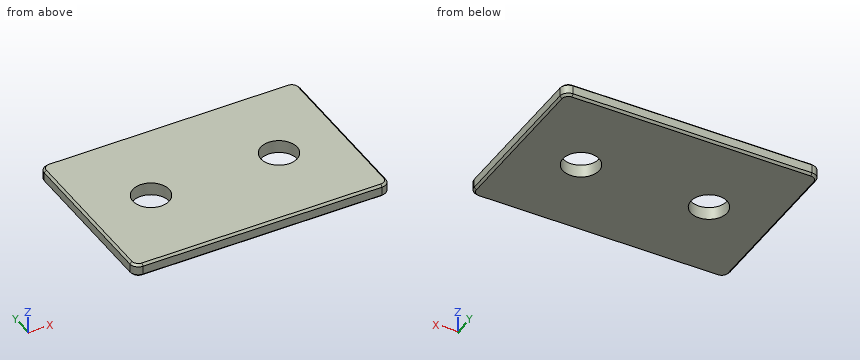
from build123d import *

# Parameters (mm, degrees)
SZKIC1_W                    = 60
SZKIC1_H                    = 40
DODANIE_WYCI_GNI_CIE1_DEPTH = 3
OTW_R_GWINTOWANY_M101_D     = 8.5
OTW_R_GWINTOWANY_M101_DEPTH = 27.5
OTW_R_GWINTOWANY_M101_TIP   = 2.553657631
ZAOKR_GLENIE1_R             = 2
SFAZOWANIE1_SIZE            = 0.5


with BuildPart() as part:
    # Szkic1 → Dodanie-wyciągnięcie1 (new body)
    with BuildSketch(Plane.XY):
        with Locations((30, 20)):
            Rectangle(SZKIC1_W, SZKIC1_H)
    extrude(amount=DODANIE_WYCI_GNI_CIE1_DEPTH)

    # Otwór gwintowany M101
    with Locations(Plane.XY.offset(3)):
        with Locations((15, 20), (45, 20)):
            Hole(OTW_R_GWINTOWANY_M101_D / 2, depth=OTW_R_GWINTOWANY_M101_DEPTH)
            with Locations((0, 0, -(OTW_R_GWINTOWANY_M101_DEPTH + OTW_R_GWINTOWANY_M101_TIP / 2))):  # 118° drill point
                Cone(0, OTW_R_GWINTOWANY_M101_D / 2, OTW_R_GWINTOWANY_M101_TIP, mode=Mode.SUBTRACT)

    # Zaokrąglenie1
    zaokr_glenie1_edges = [part.edges().sort_by_distance(p)[0] for p in [
        (0, 40, 1.5),
        (60, 40, 1.5),
        (60, 0, 1.5),
        (0, 0, 1.5),
    ]]
    fillet(zaokr_glenie1_edges, radius=ZAOKR_GLENIE1_R)

    # Sfazowanie1
    sfazowanie1_edges = [part.edges().sort_by_distance(p)[0] for p in [
        (60, 20, 0),
        (60, 20, 3),
        (0, 20, 0),
        (30, 40, 0),
        (30, 0, 0),
        (59.414213562, 39.414213562, 0),
        (0.585786438, 39.414213562, 0),
        (0.585786438, 0.585786438, 0),
        (59.414213562, 0.585786438, 0),
        (30, 0, 3),
        (0, 20, 3),
        (30, 40, 3),
        (59.414213562, 39.414213562, 3),
        (0.585786438, 39.414213562, 3),
        (0.585786438, 0.585786438, 3),
        (59.414213562, 0.585786438, 3),
    ]]
    chamfer(sfazowanie1_edges, length=SFAZOWANIE1_SIZE)


solid = part.part
Can you work these out from the model? Positions are in its coordinate system, mm. Coordinates: 2 decimals unless noted, no trailing zeros. Order: outer loops, then holes, each group sorted by start corner. A loop starts at its lowest first (then second) coordinate and runs counter-clockwise, first axis right, second up. Notation, with made-up numbers: (-18.5, -1.75) - (13.5, -1.75) arc R33 cw to (13.5, 31.25) - close; hole circle Ø3 at (50, -19). An arc over 180 degrees is marked (long way). Answer as a JSON object with one key per item and string values. Group by question number.
Q1. Imagine slicing it at B-B (y = 20). Please give me the cut outline in (x, z).
Q2. Imagine slicing it at D-D (x = 46). Please give me the cut outline in (y, z).
Q3. Imagine slicing it at C-C (z = 1.55). Please give me the cut outline in (x, y), and give its area (3 significant figures).
Q4. Imagine slicing it at A-A (x = 15). Please give me the cut outline in (y, z).
Q5. I need wall thicknesses on line 1 (Y direction, x = 15, z = 1.75); line 2 (X direction, y = 20.5, z = 2.15); line 3 (X direction, y = 23, z = 0.1). Which ranges of each line are inside material? Lowest first, please. Write a range as from..to.
Q6. Will this pin go through, and if not, where does the flat tip stop? P1, Ø7.5, axis at x = 45, y = 20, coming from the +Z side.
Determined:
{
 "1": {"outline": "(0, 0.5) - (0.5, 0) - (10.75, 0) - (10.75, 3) - (0.5, 3) - (0, 2.5) - close; (19.25, 0) - (40.75, 0) - (40.75, 3) - (19.25, 3) - close; (49.25, 0) - (59.5, 0) - (60, 0.5) - (60, 2.5) - (59.5, 3) - (49.25, 3) - close"},
 "2": {"outline": "(0, 0.5) - (0.5, 0) - (15.87, 0) - (15.87, 3) - (0.5, 3) - (0, 2.5) - close; (24.13, 0) - (39.5, 0) - (40, 0.5) - (40, 2.5) - (39.5, 3) - (24.13, 3) - close"},
 "3": {"outline": "(0, 2) arc R2 ccw to (2, 0) - (58, 0) arc R2 ccw to (60, 2) - (60, 38) arc R2 ccw to (58, 40) - (2, 40) arc R2 ccw to (0, 38) - close; hole circle Ø8.5 at (15, 20); hole circle Ø8.5 at (45, 20)", "area": "2,280 mm2"},
 "4": {"outline": "(0, 0.5) - (0.5, 0) - (15.75, 0) - (15.75, 3) - (0.5, 3) - (0, 2.5) - close; (24.25, 0) - (39.5, 0) - (40, 0.5) - (40, 2.5) - (39.5, 3) - (24.25, 3) - close"},
 "5": {"line 1": "y = 0..15.75, 24.25..40", "line 2": "x = 0..10.78, 19.22..40.78, 49.22..60", "line 3": "x = 0.4..11.99, 18.01..41.99, 48.01..59.6"},
 "6": {"P1": "passes through"}
}
